Geometry check sheet. Reference: the model listing, model coordinates, mm. A direction names the side the tool comes from. Round coordinates to 2 decimals unless told otherwise and drop trailing zeros. Write each loop counter-clockwise with the first axis right and the second up, starting at its lowest first coordinate (ties: lowest second). Pieces come first, ordered by that corner, then holes. Notation, with made-up numbers: (46, -33.75) -> (69, -33.75) arc R4 ccw to (69, -29.75) -> close; hole circle Ø8 at (26.5, 9). An arc over 180 degrees is marked (long way). Return JSON: item names as keys, results as strings. Group by question number.
from build123d import *

# Parameters (mm, degrees)
SKETCH1_R                = 47.5
SKETCH1_R_2              = 45
EXTRUDE_THIN1_DEPTH      = 20
BOSS_EXTRUDE1_REACH      = 98.852
BOSS_EXTRUDE1_END_RADIUS = 47.5
SKETCH2_W                = 2
SKETCH2_H                = 32.3
SKETCH3_W                = 12.2
SKETCH3_H                = 4.65
SKETCH3_R                = 1.1
BOSS_EXTRUDE2_DEPTH      = 2.5
SKETCH4_W                = 12.2
SKETCH4_H                = 23
CUT_EXTRUDE1_DEPTH       = 98.183602012


with BuildPart() as part:
    # Sketch1 → Extrude-Thin1 (new, symmetric)
    with BuildSketch(Plane(origin=(0, 0, 0), x_dir=(1, 0, 0), z_dir=(0, 1, 0))):
        Circle(SKETCH1_R)
        Circle(SKETCH1_R_2, mode=Mode.SUBTRACT)
    extrude(amount=EXTRUDE_THIN1_DEPTH, both=True)

    # Boss-Extrude1: up to this cylinder (the profile starts inside it)
    boss_extrude1_end = Plane(origin=(0, -5.4, 0), z_dir=(0, -1, 0)) * Cylinder(BOSS_EXTRUDE1_END_RADIUS, 293.704, mode=Mode.PRIVATE)
    # Sketch2 → Boss-Extrude1 (add, up to the surface)
    with BuildSketch(Plane.XY.offset(34.5), mode=Mode.PRIVATE) as boss_extrude1_sk1:
        with Locations((-7.1, -5.4)):
            Rectangle(SKETCH2_W, SKETCH2_H)
    boss_extrude1_tool1 = extrude(boss_extrude1_sk1.sketch, amount=BOSS_EXTRUDE1_REACH, mode=Mode.PRIVATE) & boss_extrude1_end
    add(boss_extrude1_tool1.solids().sort_by_distance((-7.1, -5.4, 34.5))[0])
    # Sketch2 → Boss-Extrude1 (add, up to the surface)
    with BuildSketch(Plane.XY.offset(34.5), mode=Mode.PRIVATE) as boss_extrude1_sk2:
        with Locations((7.1, -5.4)):
            Rectangle(SKETCH2_W, SKETCH2_H)
    boss_extrude1_tool2 = extrude(boss_extrude1_sk2.sketch, amount=BOSS_EXTRUDE1_REACH, mode=Mode.PRIVATE) & boss_extrude1_end
    add(boss_extrude1_tool2.solids().sort_by_distance((7.1, -5.4, 34.5))[0])

    # Sketch3 → Boss-Extrude2 (add)
    # profile 1 of 2: a face of its own
    with BuildSketch(Plane.XY.offset(34.5)):
        with Locations((0, -19.225)):
            Rectangle(SKETCH3_W, SKETCH3_H)
        with Locations((0, -19.55)):
            Circle(SKETCH3_R, mode=Mode.SUBTRACT)
    # profile 2 of 2: a face of its own
    with BuildSketch(Plane.XY.offset(34.5)):
        with Locations((0, 8.425)):
            Rectangle(SKETCH3_W, SKETCH3_H)
        with Locations(Location((0, 8.75, 0), (0, 0, 180))):
            Circle(SKETCH3_R, mode=Mode.SUBTRACT)
    extrude(amount=BOSS_EXTRUDE2_DEPTH)

    # Sketch4 → Cut-Extrude1 (cut, through all)
    with BuildSketch(Plane.XY.offset(34.5)):
        with Locations((0, -5.4)):
            Rectangle(SKETCH4_W, SKETCH4_H)
    extrude(amount=CUT_EXTRUDE1_DEPTH, mode=Mode.SUBTRACT)


solid = part.part
1) Sectioned sample at C-C on y = -2. Enter the section's corners in (x, z) (3 decimals).
2) Sectioned sample at D-D on x = 3.5. Enter the section's corners in (y, z).
3) Go/stop test with flat-tipped pins: P1, Ø5, axis at y = -14.5, z = 4, coming from the -X side; P2, Ø2, axis at y = 4.5, z = 30.5, coming from the -X side; P3, Ø8, axis at x = 11, y = 9.5, coming from the +Z side. Record where each tip stops, or that it passes through.
4) Material ranges on probe 1 along Y at (x, z) = (0, 36); probe 2 along X at (y, z) = (8.75, 35.2); probe 3 along X at (y, z) = (8.75, 36), recorded low to high. Write a range as [from, to].
5) Mould release check, pull along Y, two halves, no side actions. Record for faces 1 (the face through (-7, -5, 34.5)), 2 (the face through (-0.1, -21.55, 36.5)), 3 (the face through (0.238, 9.824, 35.732)): +Y half, -Y half, draft (parallel to the pull), parting line (faces both ways), or undercut.
6) Sectioned sample at B-B on x = 27. Enter the section's corners in (y, z), and give its area (3 significant figures).
7) Tool access check on faces 4 (the face through (0, 7, 37)), 5 (the face through (6.1, -6, 41)), 6 (the face through (0, -20, 46)). Record the directions out of +Z, -Z, +X, -X, +Y, -Y that give a thin tool (end or side, any length) a straight path to the whole face; none if there is none.
8) Sectioned sample at A-A on z = 0. Enter the section's corners in (x, y).
Evaluation:
{
 "1": {"outline": "(-8.1, 34.5) -> (-6.1, 34.5) -> (-6.1, 47.107) arc R47.5 ccw (long way) to (6.1, 47.107) -> (6.1, 34.5) -> (8.1, 34.5) -> (8.1, 44.265) arc R45 cw (long way) to (-8.1, 44.265) -> close"},
 "2": {"outline": "(-21.55, 34.5) -> (-16.9, 34.5) -> (-16.9, 37) -> (-21.55, 37) -> close; (-20, -47.37) -> (20, -47.37) -> (20, -44.86) -> (-20, -44.86) -> close; (-20, 44.86) -> (-16.9, 44.86) -> (-16.9, 47.37) -> (-20, 47.37) -> close; (6.1, 34.5) -> (10.75, 34.5) -> (10.75, 37) -> (6.1, 37) -> close; (6.1, 44.86) -> (20, 44.86) -> (20, 47.37) -> (6.1, 47.37) -> close"},
 "3": {"P1": "stops at x = -47.48", "P2": "stops at x = -37.23", "P3": "stops at z = 46.98"},
 "4": {"probe 1": "y = [-21.55, -20.65], [-18.45, -16.9], [6.1, 7.65], [9.85, 10.75]", "probe 2": "x = [-31.89, -28.03], [-8.1, -1.1], [1.1, 8.1], [28.03, 31.89]", "probe 3": "x = [-30.99, -27], [-8.1, -1.1], [1.1, 8.1], [27, 30.99]"},
 "5": {"face 1": "draft", "face 2": "-Y half", "face 3": "undercut"},
 "6": {"outline": "(-20, -39.08) -> (20, -39.08) -> (20, -36) -> (-20, -36) -> close; (-20, 36) -> (20, 36) -> (20, 39.08) -> (-20, 39.08) -> close", "area": "246 mm2"},
 "7": {"face 4": "+Y, -Y", "face 5": "none", "face 6": "+Z, -Y"},
 "8": {"outline": "(-47.5, -20) -> (-45, -20) -> (-45, 20) -> (-47.5, 20) -> close; (45, -20) -> (47.5, -20) -> (47.5, 20) -> (45, 20) -> close"}
}
